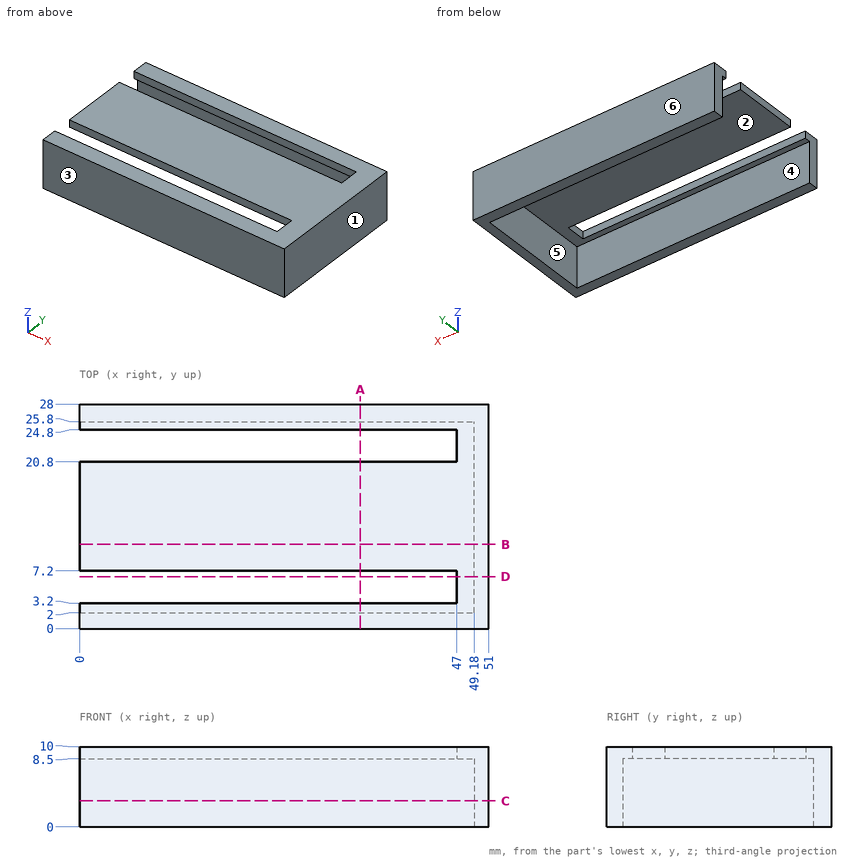
Study the drawing (mm; zero at the part's minimum x, y, z) and answer. A direction names the side the tool comes from. Round coordinates to 2 decimals unless told otherwise and drop trailing zeros. Write each loop counter-clockwise with the first axis right and the second up, starting at its lowest first coordinate (ties: lowest second). Pieces come first, ordered by that corner, then holes.
1) Given pin 1 Ø1.2 at (y, z) = (23.5, 9.5) entering from -X; pin 2 Ø6 at (x, y) = (11.5, 10.5) entering from -Z; pin 3 Ø1.2 at (x, z) = (31, 9) entering from -Y; pin 4 Ø1.5 at (y, z) = (11, 3.5) entering from -X, each flat-ended and moving along its own axis, determine where each tip first touches the part or whether it passes through.
2) A cutting plane is placed at C-C (z = 3.25). Give the vertices of the cut face in (x, y), plus the area to 3 significant figures.
3) A cutting plane is placed at B-B (y = 10.5). Give the vertices of the cut face in (x, z).
4) A tool of negligible diameter and unlimited length cuts with its end or side. For the marked faces 5 and 6, from which of +Z, -Z, +X, -X, +Y, -Y can it reach the whole face along a straight path? Write none if from no direction.
5) A cutting plane is placed at A-A (x = 35). Give the vertices of the cut face in (y, z), plus the area to 3 significant figures.
6) Straight lines are drawn through the part: line 1 (Y direction, x = 17, z = 9.75); line 2 (Y direction, x = 10, z = 1.25); line 3 (X direction, y = 23.75, z = 7.75). For each, find the intervals that lie inside material, in ascending order.
7) A cutting plane is placed at D-D (y = 6.5). Give the vertices of the cut face in (x, z), plus the area to 3 significant figures.
8) The mould has two halves that part along Y. Classify the marked faces 1, 2, 3 and 4: pulls with the +Y half, pulls with the -Y half, needs draft (parallel to the pull), parting line crosses it, or undercut.
Completed:
1. pin 1: stops at x = 47
1. pin 2: stops at z = 8.5
1. pin 3: stops at y = 0
1. pin 4: stops at x = 49.18
2. outline: (0, 0) - (51, 0) - (51, 28) - (0, 28) - (0, 25.8) - (49.18, 25.8) - (49.18, 2) - (0, 2) - close
2. area: 258 mm2
3. outline: (0, 8.5) - (49.18, 8.5) - (49.18, 0) - (51, 0) - (51, 10) - (0, 10) - close
4. face 5: -Z, -X
4. face 6: +Z, -Z, +X, -X, +Y
5. outline: (0, 0) - (2, 0) - (2, 8.5) - (3.2, 8.5) - (3.2, 10) - (0, 10) - close; (7.2, 8.5) - (20.8, 8.5) - (20.8, 10) - (7.2, 10) - close; (24.8, 8.5) - (25.8, 8.5) - (25.8, 0) - (28, 0) - (28, 10) - (24.8, 10) - close
5. area: 65.7 mm2
6. line 1: y = 0 to 3.2, 7.2 to 20.8, 24.8 to 28
6. line 2: y = 0 to 2, 25.8 to 28
6. line 3: x = 49.18 to 51
7. outline: (47, 8.5) - (49.18, 8.5) - (49.18, 0) - (51, 0) - (51, 10) - (47, 10) - close
7. area: 21.5 mm2
8. face 1: needs draft
8. face 2: undercut
8. face 3: pulls with the -Y half
8. face 4: undercut
